Design review of the part built by this model. Coordinates are the model's own, in mm. A direction names the side the tool comes from. Coordinates: 2 decimals unless noted, no trailing zeros. Loops run counter-clockwise (first coordinate to the right, second up) from the corner with the lowest first, then second, coordinate; pieces in that order, holes last. Notation, with made-up numbers: (-1, 87.5) -> (16, 87.5) arc R14 ccw to (16, 110.5) -> close; hole circle Ø5 at (14.25, -24.75). An arc over 180 degrees is marked (long way). One line per item, written item: value. Start each with the question number.
1. Insertion check: pin 1 (5 mm diameter, centred on x = 18.5, y = 7.5, fed in from +Z); pin 2 (1.2 mm diameter, centred on x = 79, y = 0.5, fed in from +Z); pin 3 (1 mm diameter, centred on y = 5.5, z = -0.5, fed in from -X); pin 4 (4.5 mm diameter, centred on x = -2, z = -4, fed in from -Y). Each pin has a flat end and moves straight along its axis. Give the tip position at first contact, or say it passes through.
2. Add section D-D on z = -83. Write out the cut boundary in (x, y).
3. Machinability: for faces 1 (the flat face through (154, 10, 0)), 2 (the flat face through (6, 1, -13.707)), 3 (the flat face through (6, 11, -1.5)), 4 (the flat face through (75.5, 1, -9)), 5 (the flat face through (44, 10, -100)), which of the approach directions +Z, -Z, +X, -X, +Y, -Y give a long, thin tool a straight path to every point of the face, cutting with its end or side? Answer none if there is none.
4. Add section C-C on z = -4. Write out the cut boundary in (x, y).
5. For probe 1 along X at (y, z) = (8.75, -96); probe 2 along Z at (x, y) = (162, 13.25); probe 3 along Z at (x, y) = (153, 12), list the stretches that pass through material, from the lowest coordinate up.
6. Add section B-B on y = 12. Give the number of separate pieces and of enclosed holes in the cut face, plus the area to 3 significant figures.
7. Add section A-A on x = 16. Write out the cut boundary in (y, z), plus the area to 3 significant figures.
8. Draft analysis for pull direction Z (two halves, no side actions). For faces 6 (the flat face through (49, 10, 0)), 7 (the flat face through (93.5, 8, -99)), 8 (the flat face through (146, 11, -98.5)), 9 (the flat face through (158.826, 11, -9)), state which applies: pulls with the +Z half, pulls with the -Z half, needs draft (parallel to the pull), parting line crosses it, or undercut.
```python
from build123d import *

# Parameters (mm, degrees)
SKETCH1_W           = 160
SKETCH1_H           = 100
BOSS_EXTRUDE1_DEPTH = 1.5
SKETCH2_W           = 160
SKETCH2_H           = 100
SKETCH2_W_2         = 157
SKETCH2_H_2         = 97
BOSS_EXTRUDE2_DEPTH = 20
FILLET1_R           = 2
SKETCH4_W           = 15
SKETCH4_H           = 21
CUT_EXTRUDE1_DEPTH  = 190.73665961
SKETCH5_W           = 69
SKETCH5_H           = 26.5
CUT_EXTRUDE2_DEPTH  = 190.73665961
SKETCH6_W           = 11.5
SKETCH6_H           = 43
CUT_EXTRUDE3_DEPTH  = 190.73665961
CUT_EXTRUDE5_DEPTH  = 10
FILLET2_R           = 2
SKETCH10_W          = 13
SKETCH10_H          = 2
CUT_EXTRUDE6_DEPTH  = 20
FILLET4_R           = 2
SKETCH11_W          = 25
SKETCH11_H          = 10
CUT_EXTRUDE7_DEPTH  = 20
FILLET5_R           = 2
SKETCH12_W          = 8
SKETCH12_H          = 8
SKETCH12_R          = 1.65
BOSS_EXTRUDE3_DEPTH = 20
FILLET6_R           = 2
SKETCH14_W          = 24
SKETCH14_H          = 64.876727664
CUT_EXTRUDE8_DEPTH  = 22
SKETCH16_W          = 24
SKETCH16_H          = 5
CUT_EXTRUDE9_DEPTH  = 20
FILLET8_R           = 2
SKETCH18_W          = 24
SKETCH18_H          = 5
CUT_EXTRUDE10_DEPTH = 20
FILLET9_R           = 2


with BuildPart() as part:
    # Sketch1 → Boss-Extrude1 (new body)
    with BuildSketch(Plane(origin=(0, 0, 0), x_dir=(1, 0, 0), z_dir=(0, 1, 0))):
        with Locations((80, 50)):
            Rectangle(SKETCH1_W, SKETCH1_H)
    extrude(amount=BOSS_EXTRUDE1_DEPTH)

    # Sketch2 → Boss-Extrude2 (add)
    with BuildSketch(Plane(origin=(0, 0, 0), x_dir=(1, 0, 0), z_dir=(0, 1, 0))):
        with Locations((80, 50)):
            Rectangle(SKETCH2_W, SKETCH2_H)
        with Locations((80.326409395, 50)):
            Rectangle(SKETCH2_W_2, SKETCH2_H_2, mode=Mode.SUBTRACT)
    extrude(amount=BOSS_EXTRUDE2_DEPTH)

    # Fillet1
    fillet1_edges = [part.edges().sort_by_distance(p)[0] for p in [
        (0, 10, -100),
        (160, 10, -100),
        (160, 10, 0),
        (0, 10, 0),
    ]]
    fillet(fillet1_edges, radius=FILLET1_R)

    # Sketch4 → Cut-Extrude1 (cut, through all)
    with BuildSketch(Plane.XZ):
        with Locations((126, -89.5)):
            Rectangle(SKETCH4_W, SKETCH4_H)
    extrude(amount=-CUT_EXTRUDE1_DEPTH, mode=Mode.SUBTRACT)

    # Sketch5 → Cut-Extrude2 (cut, through all)
    with BuildSketch(Plane.XZ):
        with Locations((110, -13.25)):
            Rectangle(SKETCH5_W, SKETCH5_H)
    extrude(amount=-CUT_EXTRUDE2_DEPTH, mode=Mode.SUBTRACT)

    # Sketch6 → Cut-Extrude3 (cut, through all)
    with BuildSketch(Plane.XZ):
        with Locations((154.25, -32.5)):
            Rectangle(SKETCH6_W, SKETCH6_H)
    extrude(amount=-CUT_EXTRUDE3_DEPTH, mode=Mode.SUBTRACT)

    # Sketch9 → Cut-Extrude5 (cut)
    with BuildSketch(Plane.XZ):
        with BuildLine():
            Line((134.539408017, -26.5), (123.460591983, -26.5))
            ThreePointArc((123.460591983, -26.5), (129, -32.039408017), (134.539408017, -26.5))
        make_face()
        with BuildLine():
            Line((96.539, -26.5), (85.461, -26.5))
            ThreePointArc((85.461, -26.5), (91, -32.039), (96.539, -26.5))
        make_face()
    extrude(amount=-CUT_EXTRUDE5_DEPTH, mode=Mode.SUBTRACT)

    # Fillet2
    fillet2_edges = [part.edges().sort_by_distance(p)[0] for p in [
        (85.461, 0.75, -26.5),
        (96.539, 0.75, -26.5),
        (123.460591983, 0.75, -26.5),
        (134.539408017, 0.75, -26.5),
    ]]
    fillet(fillet2_edges, radius=FILLET2_R)

    # Sketch10 → Cut-Extrude6 (cut)
    with BuildSketch(Plane.XZ):
        with Locations((16.208817875, -1)):
            Rectangle(SKETCH10_W, SKETCH10_H)
    extrude(amount=-CUT_EXTRUDE6_DEPTH, mode=Mode.SUBTRACT)

    # Fillet4
    fillet4_edges = [part.edges().sort_by_distance(p)[0] for p in [
        (148.5, 0.75, -54),
        (148.5, 0.75, -11),
        (118.5, 0.75, -79),
        (133.5, 0.75, -79),
    ]]
    fillet(fillet4_edges, radius=FILLET4_R)

    # Sketch11 → Cut-Extrude7 (cut)
    with BuildSketch(Plane.XZ):
        with Locations((106, -95)):
            Rectangle(SKETCH11_W, SKETCH11_H)
    extrude(amount=-CUT_EXTRUDE7_DEPTH, mode=Mode.SUBTRACT)

    # Fillet5
    fillet5_edges = [part.edges().sort_by_distance(p)[0] for p in [
        (118.5, 0.75, -90),
        (93.5, 0.75, -90),
    ]]
    fillet(fillet5_edges, radius=FILLET5_R)

    # Sketch12 → Boss-Extrude3 (add)
    # profile 1 of 4: a face of its own
    with BuildSketch(Plane.XZ):
        with Locations((-2, -4)):
            Rectangle(SKETCH12_W, SKETCH12_H)
        with Locations(Location((-2, -4, 0), (0, 0, 90))):
            Circle(SKETCH12_R, mode=Mode.SUBTRACT)
    # profile 2 of 4: a face of its own
    with BuildSketch(Plane.XZ):
        with Locations((162, -96)):
            Rectangle(SKETCH12_W, SKETCH12_H)
        with Locations(Location((162, -96, 0), (0, 0, 270))):
            Circle(SKETCH12_R, mode=Mode.SUBTRACT)
    # profile 3 of 4: a face of its own
    with BuildSketch(Plane.XZ):
        with Locations((162, -4)):
            Rectangle(SKETCH12_W, SKETCH12_H)
        with Locations(Location((162, -4, 0), (0, 0, 270))):
            Circle(SKETCH12_R, mode=Mode.SUBTRACT)
    # profile 4 of 4: a face of its own
    with BuildSketch(Plane.XZ):
        with Locations((-2, -96)):
            Rectangle(SKETCH12_W, SKETCH12_H)
        with Locations(Location((-2, -96, 0), (0, 0, 90))):
            Circle(SKETCH12_R, mode=Mode.SUBTRACT)
    extrude(amount=-BOSS_EXTRUDE3_DEPTH)

    # Fillet6
    fillet6_edges = [part.edges().sort_by_distance(p)[0] for p in [
        (160, 10, -92),
        (166, 10, -92),
        (166, 10, -100),
        (166, 10, -8),
        (160, 10, -8),
        (166, 10, 0),
        (0, 10, -8),
        (-6, 10, -8),
        (-6, 10, 0),
        (-6, 10, -92),
        (0, 10, -92),
        (-6, 10, -100),
    ]]
    fillet(fillet6_edges, radius=FILLET6_R)

    # Sketch14 → Cut-Extrude8 (cut)
    with BuildSketch(Plane.XZ):
        with Locations((12, -51.145467828)):
            Rectangle(SKETCH14_W, SKETCH14_H)
    extrude(amount=-CUT_EXTRUDE8_DEPTH, mode=Mode.SUBTRACT)

    # Sketch16 → Cut-Extrude9 (cut)
    with BuildSketch(Plane.XZ):
        with Locations((12, -86.08383166)):
            Rectangle(SKETCH16_W, SKETCH16_H)
    extrude(amount=-CUT_EXTRUDE9_DEPTH, mode=Mode.SUBTRACT)

    # Fillet8
    fillet8_edges = [part.edges().sort_by_distance(p)[0] for p in [
        (24, 0.75, -88.58383166),
    ]]
    fillet(fillet8_edges, radius=FILLET8_R)

    # Sketch18 → Cut-Extrude10 (cut)
    with BuildSketch(Plane.XZ):
        with Locations((12, -16.207103996)):
            Rectangle(SKETCH18_W, SKETCH18_H)
    extrude(amount=-CUT_EXTRUDE10_DEPTH, mode=Mode.SUBTRACT)

    # Fillet9
    fillet9_edges = [part.edges().sort_by_distance(p)[0] for p in [
        (24, 0.75, -13.707103996),
    ]]
    fillet(fillet9_edges, radius=FILLET9_R)


solid = part.part
```
Worked answers:
1. pin 1: stops at z = -98.5
1. pin 2: stops at z = -26.5
1. pin 3: stops at x = -5.73
1. pin 4: stops at y = 0
2. outline: (24, 0) -> (118.5, 0) -> (118.5, 1.5) -> (24, 1.5) -> close; (133.5, 0) -> (160, 0) -> (160, 20) -> (158.83, 20) -> (158.83, 1.5) -> (133.5, 1.5) -> close
3. face 1: +Z, +X, -X, +Y, -Y
3. face 2: -X, +Y, -Y
3. face 3: +Y
3. face 4: +Z, +Y, -Y
3. face 5: -Z, +X, -X, +Y, -Y
4. outline: (-6, 0) -> (-3.65, 0) -> (-3.65, 20) -> (-6, 20) -> close; (-0.35, 0) -> (75.5, 0) -> (75.5, 1.5) -> (2, 1.5) -> (2, 20) -> (-0.35, 20) -> close; (144.5, 0) -> (160.35, 0) -> (160.35, 20) -> (158, 20) -> (158, 1.5) -> (144.5, 1.5) -> close; (163.65, 0) -> (166, 0) -> (166, 20) -> (163.65, 20) -> close
5. probe 1: x = -6 to -3.65, -0.35 to 2, 158 to 160.35, 163.65 to 166
5. probe 2: z = -100 to -97.65, -94.35 to -92, -8 to -5.65, -2.35 to 0
5. probe 3: z = -100 to -98.5, -1.5 to 0
6. separate pieces: 5
6. enclosed holes: 4
6. area: 568 mm²
7. outline: (0, -100) -> (20, -100) -> (20, -98.5) -> (1.5, -98.5) -> (1.5, -88.58) -> (0, -88.58) -> close; (0, -13.71) -> (1.5, -13.71) -> (1.5, -2) -> (0, -2) -> close
7. area: 62.4 mm²
8. face 6: pulls with the +Z half
8. face 7: needs draft
8. face 8: undercut
8. face 9: undercut
